from build123d import *

# Parameters (mm, degrees)
SKETCH_1_R          = 6.25
SKETCH_1_R_2        = 2.75
EXTRUDE_1_DEPTH     = 24.5
SKETCH_1_3_R        = 1.5
SKETCH_1_3_W        = 12.5
SKETCH_1_3_H        = 5.05
EXTRUDE_2_DEPTH     = 19.5
SKETCH_1_4_R        = 1.5
SKETCH_1_4_W        = 12.5
SKETCH_1_4_H        = 5.05
CUT_EXTRUDE_1_DEPTH = 17
SKETCH_1_5_R        = 6.25
SKETCH_1_5_R_2      = 2.75
EXTRUDE_3_DEPTH     = 28.5
SKETCH_1_6_R        = 2.75
EXTRUDE_4_DEPTH     = 32


with BuildPart() as part:
    # Sketch 1 → Extrude 1 (new body)
    # profile 1 of 5: a face of its own
    with BuildSketch(Plane.XY):
        with BuildLine():
            Line((-6.25, 4.999999984), (-6.25, -11.25))
            Line((-6.25, -11.25), (6.25, -11.25))
            Line((6.25, -11.25), (6.25, 5))
            ThreePointArc((6.25, 5), (8e-09, -1.25), (-6.25, 4.999999984))
        make_face()
    # profile 2 of 5: a face of its own
    with BuildSketch(Plane.XY):
        with Locations((0, 5)):
            Circle(SKETCH_1_R)
        with Locations((0, 5)):
            Circle(SKETCH_1_R_2, mode=Mode.SUBTRACT)
    # profile 3 of 5: a face of its own
    with BuildSketch(Plane.XY):
        with Locations((0, 5)):
            Circle(SKETCH_1_R_2)
    # profile 4 of 5: a face of its own
    with BuildSketch(Plane.XY):
        with BuildLine():
            Line((-6.25, 11.25), (-6.25, 4.999999984))
            ThreePointArc((-6.25, 4.999999984), (-4.419417379, 9.419417386), (2.6e-08, 11.25))
            Line((2.6e-08, 11.25), (-6.25, 11.25))
        make_face()
    # profile 5 of 5: a face of its own
    with BuildSketch(Plane.XY):
        with BuildLine():
            ThreePointArc((2.6e-08, 11.25), (4.419417392, 9.419417373), (6.25, 5))
            Line((6.25, 5), (6.25, 11.25))
            Line((6.25, 11.25), (2.6e-08, 11.25))
        make_face()
    extrude(amount=EXTRUDE_1_DEPTH)

    # Sketch 1_3 → Extrude 2 (add)
    # profile 1 of 2: a face of its own
    with BuildSketch(Plane.XY):
        Polygon((-6.25, 16.3), (-6.25, 11.25), (2.6e-08, 11.25), (6.25, 11.25), (6.25, 16.3), align=None)
        with Locations((0, 13.8)):
            Circle(SKETCH_1_3_R, mode=Mode.SUBTRACT)
    # profile 2 of 2: a face of its own
    with BuildSketch(Plane.XY):
        with Locations((0, -13.775)):
            Rectangle(SKETCH_1_3_W, SKETCH_1_3_H)
        with Locations((0, -13.8)):
            Circle(SKETCH_1_3_R, mode=Mode.SUBTRACT)
    extrude(amount=EXTRUDE_2_DEPTH)

    # Sketch 1_4 → Cut-Extrude 1 (cut)
    # profile 1 of 2: a face of its own
    with BuildSketch(Plane.XY):
        Polygon((-6.25, 16.3), (-6.25, 11.25), (2.6e-08, 11.25), (6.25, 11.25), (6.25, 16.3), align=None)
        with Locations((0, 13.8)):
            Circle(SKETCH_1_4_R, mode=Mode.SUBTRACT)
    # profile 2 of 2: a face of its own
    with BuildSketch(Plane.XY):
        with Locations((0, -13.775)):
            Rectangle(SKETCH_1_4_W, SKETCH_1_4_H)
        with Locations((0, -13.8)):
            Circle(SKETCH_1_4_R, mode=Mode.SUBTRACT)
    extrude(amount=CUT_EXTRUDE_1_DEPTH, mode=Mode.SUBTRACT)

    # Sketch 1_5 → Extrude 3 (add)
    # profile 1 of 2: a face of its own
    with BuildSketch(Plane.XY):
        with Locations((0, 5)):
            Circle(SKETCH_1_5_R)
        with Locations((0, 5)):
            Circle(SKETCH_1_5_R_2, mode=Mode.SUBTRACT)
    # profile 2 of 2: a face of its own
    with BuildSketch(Plane.XY):
        with Locations((0, 5)):
            Circle(SKETCH_1_5_R_2)
    extrude(amount=EXTRUDE_3_DEPTH)

    # Sketch 1_6 → Extrude 4 (add)
    with BuildSketch(Plane.XY):
        with Locations((0, 5)):
            Circle(SKETCH_1_6_R)
    extrude(amount=EXTRUDE_4_DEPTH)


solid = part.part
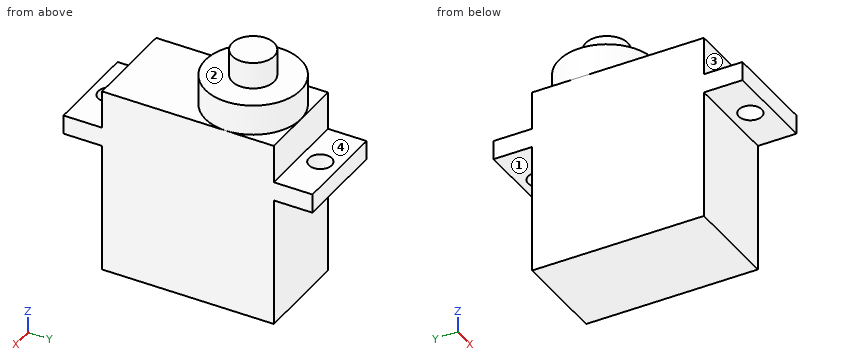
Model file for the job. Use its own axes, mm. Face numbers are marked on the shaded views. A direction names the side the tool comes from. Give positions to 0.01 mm unless a question says otherwise; leave off trailing zeros. Loops run counter-clockwise (first coordinate to the right, second up) from the corner with the lowest first, then second, coordinate; pieces in that order, holes last.
Item 1: Drill centre lines: line 1 along Y through (x, z) = (0, 18.25); line 2 along Z through (x, y) = (-2.25, -11); line 3 along Y through (x, z) = (-1, 7). Where is each one in solid material? Low to high.
Check values:
line 1: y = -16.3 to -15.3, -12.3 to 12.3, 15.3 to 16.3
line 2: z = 0 to 24.5
line 3: y = -11.25 to 11.25
Item 2: Which spindle directions (+Z, -Z, +X, -X, +Y, -Y) get a long thin tool onto all of the face, cutting with end or side? Do the marked faces 1, 2, 3 and 4. Say none if no direction does.
Check values:
face 1: -Z, +X, -X, +Y
face 2: +Z
face 3: +Z, +X, -X, -Y
face 4: +Z, +X, -X, +Y
Item 3: Slice it at C-C (y = 0). Write the cut outline in (x, z).
Check values:
outline: (-6.25, 0) - (6.25, 0) - (6.25, 24.5) - (3.75, 24.5) - (3.75, 28.5) - (-3.75, 28.5) - (-3.75, 24.5) - (-6.25, 24.5) - close
Item 4: Drop flat-ended pins along their axis: P1, Ø3, axis at x = 2, y = -1.5, coming from the +Z side; P2, Ø4, axis at x = -1, z = 6, coming from the -Y side; P3, Ø5, axis at x = 0, y = 13.8, coming from the -Z side; P4, Ø1, axis at y = -12, z = 9.5, coming from the +X side. Give the stop position or say it passes through.
Check values:
P1: stops at z = 28.5
P2: stops at y = -11.25
P3: stops at z = 17
P4: passes through
Item 5: Slice it at A-A (y = -13.8). Write the cut outline in (x, z).
Check values:
outline: (-6.25, 17) - (-1.5, 17) - (-1.5, 19.5) - (-6.25, 19.5) - close; (1.5, 17) - (6.25, 17) - (6.25, 19.5) - (1.5, 19.5) - close
Item 6: Slice it at B-B (x = -4.25). Write the cut outline in (y, z), plus the area to 3 significant figures.
Check values:
outline: (-16.3, 17) - (-11.25, 17) - (-11.25, 0) - (11.25, 0) - (11.25, 17) - (16.3, 17) - (16.3, 19.5) - (11.25, 19.5) - (11.25, 24.5) - (9.58, 24.5) - (9.58, 28.5) - (0.42, 28.5) - (0.42, 24.5) - (-11.25, 24.5) - (-11.25, 19.5) - (-16.3, 19.5) - close
area: 613 mm2
